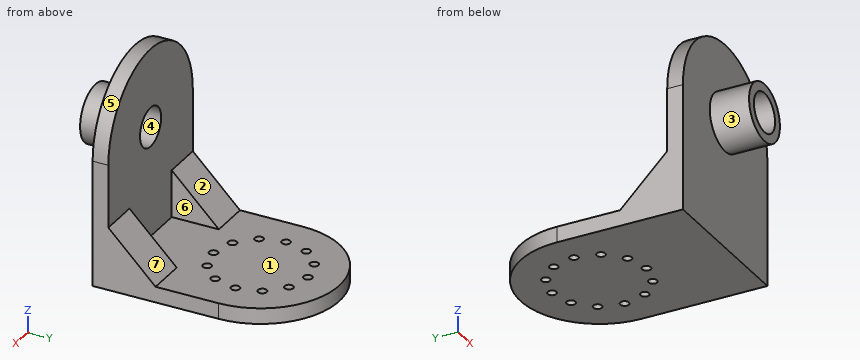
```python
from build123d import *

# Parameters (mm, degrees)
EXTRUDE_1_DEPTH     = 10
EXTRUDE_2_DEPTH     = 10
EXTRUDE_3_DEPTH     = 25
EXTRUDE_4_DEPTH     = 25
SKETCH_5_R          = 2.75
CUT_EXTRUDE_1_DEPTH = 25
SKETCH_6_R          = 18.25
SKETCH_6_R_2        = 12.5
EXTRUDE_5_DEPTH     = 25
CUT_EXTRUDE_START   = -10
SKETCH_7_R          = 12.5
CUT_EXTRUDE_2_DEPTH = 10


with BuildPart() as part:
    # 草图1 → 凸台-拉伸1 (new body)
    with BuildSketch(Plane.XY):
        with BuildLine():
            Line((-50, 0), (-50, -80))
            Line((-50, -80), (50, -80))
            Line((50, -80), (50, 0))
            ThreePointArc((50, 0), (0, 50), (-50, 0))
        make_face()
    extrude(amount=EXTRUDE_1_DEPTH)

    # 草图2 → 凸台-拉伸2 (add)
    with BuildSketch(Plane.XZ.offset(80)):
        with BuildLine():
            Line((50, 10), (50, 80))
            ThreePointArc((50, 80), (0, 130), (-50, 80))
            Line((-50, 80), (-50, 10))
            Line((-50, 10), (50, 10))
        make_face()
    extrude(amount=-EXTRUDE_2_DEPTH)

    # 草图3 → 凸台-拉伸3 (add)
    with BuildSketch(Plane.ZY.offset(50)):
        Polygon((10, -40), (40, -70), (10, -70), align=None)
    extrude(amount=-EXTRUDE_3_DEPTH)

    # 草图4 → 凸台-拉伸4 (add)
    with BuildSketch(Plane(origin=(50, 0, 0), x_dir=(0, 0, -1), z_dir=(1, 0, 0))):
        Polygon((-10, -70), (-10, -40), (-40, -70), align=None)
    extrude(amount=-EXTRUDE_4_DEPTH)

    # 草图5 → 切除-拉伸1 (cut)
    with BuildSketch(Plane.XY.offset(10)):
        with Locations((0, 30)):
            Circle(SKETCH_5_R)
        with Locations((30, 0)):
            Circle(SKETCH_5_R)
        with Locations((0, -30)):
            Circle(SKETCH_5_R)
        with Locations((-30, 0)):
            Circle(SKETCH_5_R)
        with Locations((15, 25.980762114)):
            Circle(SKETCH_5_R)
        with Locations((25.980762114, 15)):
            Circle(SKETCH_5_R)
        with Locations((15, -25.980762114)):
            Circle(SKETCH_5_R)
        with Locations((25.980762114, -15)):
            Circle(SKETCH_5_R)
        with Locations((-15, 25.980762114)):
            Circle(SKETCH_5_R)
        with Locations((-25.980762114, 15)):
            Circle(SKETCH_5_R)
        with Locations((-25.980762114, -15)):
            Circle(SKETCH_5_R)
        with Locations((-15, -25.980762114)):
            Circle(SKETCH_5_R)
    extrude(amount=-CUT_EXTRUDE_1_DEPTH, mode=Mode.SUBTRACT)

    # 草图6 → 凸台-拉伸5 (add)
    with BuildSketch(Plane.XZ.offset(80)):
        with Locations(Location((0, 80, 0), (0, 0, 90))):
            Circle(SKETCH_6_R)
        with Locations(Location((0, 80, 0), (0, 0, 270))):
            Circle(SKETCH_6_R_2, mode=Mode.SUBTRACT)
    extrude(amount=EXTRUDE_5_DEPTH)

    # 草图7 → 切除-拉伸2 (cut)
    with BuildSketch(Plane.XZ.offset(80).offset(CUT_EXTRUDE_START)):
        with Locations(Location((0, 80, 0), (0, 0, 270))):
            Circle(SKETCH_7_R)
    extrude(amount=CUT_EXTRUDE_2_DEPTH, mode=Mode.SUBTRACT)


solid = part.part
```
Could you check a few things on this model? Use its own coordinates, in mm. Face numbers are marked on the shaded views. A direction names the side the tool comes from. Coordinates: 2 decimals unless noted, no trailing zeros. Loops run counter-clockwise (first coordinate to the right, second up) from the corner with the lowest first, then second, coordinate; pieces in that order, holes last.
1) Thinking about a two-plate mould opening in X: for the marked faces 4, 5, 6 and 7, which applies, released by +X, released by -X, zero draft, split by the parting line, or undercut?
Reported:
face 4: undercut
face 5: split by the parting line
face 6: undercut
face 7: zero draft
2) Will these pins go through, and if not, where does the flat tip stop? pin 1 Ø10 at (x, z) = (-33.5, 85) entering from +Y; pin 2 Ø8 at (x, y) = (4.5, -0.5) entering from -Z; pin 3 Ø5 at (x, y) = (-15, 25.98) entering from +Z; pin 4 Ø2 at (x, z) = (12, 26.5) entering from -Y.
Reported:
pin 1: stops at y = -70
pin 2: stops at z = 0
pin 3: passes through
pin 4: stops at y = -80
3) Imagine slicing it at A-A (y = -15). List the corners of the cut face in (x, z) for me, and give its area (3 significant figures).
Reported:
outline: (-50, 0) - (-28.73, 0) - (-28.73, 10) - (-50, 10) - close; (-23.23, 0) - (23.23, 0) - (23.23, 10) - (-23.23, 10) - close; (28.73, 0) - (50, 0) - (50, 10) - (28.73, 10) - close
area: 890 mm2
4) Which directions (+Z, -Z, +X, -X, +Y, -Y) give clear straight access to the entire face, cutting with the end or side of a thin tool? Please do the marked faces 1, 2 and 3.
Reported:
face 1: +Z, +Y
face 2: +Z, +X, -X, +Y
face 3: -Y
5) Please list where these lines run through material, in increasing order: line 1 along Y through (x, z) = (0, 5.5); line 2 along X through (y, z) = (-60, 11); line 3 along Y through (x, z) = (-15, 6).
Reported:
line 1: y = -80 to -32.75, -27.25 to 27.25, 32.75 to 50
line 2: x = -50 to -25, 25 to 50
line 3: y = -80 to -28.73, -23.23 to 23.23, 28.73 to 47.7
6) Imagine slicing it at D-D (y = -52). List the corners of the cut face in (x, z) for me.
Reported:
outline: (-50, 0) - (50, 0) - (50, 22) - (25, 22) - (25, 10) - (-25, 10) - (-25, 22) - (-50, 22) - close
7) Imagine slicing it at C-C (x = -15). List the corners of the cut face in (y, z) for me, and give its area (3 significant figures).
Reported:
outline: (-105, 69.6) - (-80, 69.6) - (-80, 0) - (-28.73, 0) - (-28.73, 10) - (-70, 10) - (-70, 127.7) - (-80, 127.7) - (-80, 90.4) - (-105, 90.4) - close; (-23.23, 0) - (23.23, 0) - (23.23, 10) - (-23.23, 10) - close; (28.73, 0) - (47.7, 0) - (47.7, 10) - (28.73, 10) - close
area: 2,860 mm2
8) Imagine slicing it at B-B (z = 88). List the corners of the cut face in (x, y) for me.
Reported:
outline: (-49.36, -80) - (-16.4, -80) - (-16.4, -105) - (-9.6, -105) - (-9.6, -70) - (-49.36, -70) - close; (9.6, -105) - (16.4, -105) - (16.4, -80) - (49.36, -80) - (49.36, -70) - (9.6, -70) - close
